The listing builds one solid part. Answer for the finished solid, in the listing's coordinates (mm). Face numbers are marked on the shaded views. A direction names the side the tool comes from. Give positions to 0.01 mm unless a question says otherwise; leave off trailing zeros. Order: outer loops, then holes, each group sorted by start corner. A loop starts at its lowest first (then second) coordinate and runs counter-clockwise, first axis right, second up.
```python
from build123d import *

# Parameters (mm, degrees)
EXTRUDE_1_DEPTH      = 25
CUT_EXTRUDE_1_REACH  = 113.383
SKETCH_2_R           = 3.2
CUT_EXTRUDE_2_REACH  = 113.383
SKETCH_3_R           = 3.2
SKETCH_14_W          = 22.5
SKETCH_14_H          = 2.5
SKETCH_14_W_2        = 2.5
SKETCH_14_H_2        = 22.5
CUT_EXTRUDE_12_DEPTH = 25
SKETCH_5_W           = 20.4
SKETCH_5_H           = 20.4
CUT_EXTRUDE_7_DEPTH  = 25
EXTRUDE_2_DEPTH      = 10
SKETCH_10_R          = 3.2
CUT_EXTRUDE_8_DEPTH  = 17.1
SKETCH_11_R          = 5.25
CUT_EXTRUDE_9_DEPTH  = 12.1
SKETCH_12_R          = 3.2
CUT_EXTRUDE_10_DEPTH = 17.1
SKETCH_13_R          = 5.25
CUT_EXTRUDE_11_DEPTH = 12.1
FILLET_2_R           = 2.5
FILLET_3_R           = 15
FILLET_5_R           = 2.5


with BuildPart() as part:
    # 스케치1 → 보스-돌출1 (new body)
    with BuildSketch(Plane(origin=(0, 0, 0), x_dir=(1, 0, 0), z_dir=(0, 1, 0))):
        Polygon((-17.5, 67.5), (-11.25, 67.5), (-11.25, 37.5), (11.25, 37.5), (11.25, 67.5), (17.5, 67.5), (17.5, -17.5), (-67.5, -17.5), (-67.5, -11.25), (-37.5, -11.25), (-37.5, 11.25), (-67.5, 11.25), (-67.5, 17.5), (-17.5, 17.5), align=None)
    extrude(amount=EXTRUDE_1_DEPTH)

    # 컷-돌출1: up to this face of the body (flat: up to its plane)
    cut_extrude_1_end = Plane(part.part.faces().sort_by_distance((-17.5, 12.5, -42.5))[0])
    # 스케치2 → 컷-돌출1 (cut, up to the picked face)
    with BuildSketch(Plane(origin=(17.5, 0, 0), x_dir=(0, 0, -1), z_dir=(1, 0, 0)), mode=Mode.PRIVATE) as cut_extrude_1_sk1:
        with Locations((60, 12.5)):
            Circle(SKETCH_2_R)
    cut_extrude_1_tool1 = split(extrude(cut_extrude_1_sk1.sketch, amount=-CUT_EXTRUDE_1_REACH, mode=Mode.PRIVATE), bisect_by=cut_extrude_1_end, keep=Keep.BOTH, mode=Mode.PRIVATE)
    # 스케치2 → 컷-돌출1 (cut, up to the picked face)
    with BuildSketch(Plane(origin=(17.5, 0, 0), x_dir=(0, 0, -1), z_dir=(1, 0, 0)), mode=Mode.PRIVATE) as cut_extrude_1_sk2:
        with Locations((45, 12.5)):
            Circle(SKETCH_2_R)
    cut_extrude_1_tool2 = split(extrude(cut_extrude_1_sk2.sketch, amount=-CUT_EXTRUDE_1_REACH, mode=Mode.PRIVATE), bisect_by=cut_extrude_1_end, keep=Keep.BOTH, mode=Mode.PRIVATE)
    add(cut_extrude_1_tool1.solids().sort_by(Axis((17.5, 12.5, -60), (-1, 0, 0)))[0], mode=Mode.SUBTRACT)
    add(cut_extrude_1_tool2.solids().sort_by(Axis((17.5, 12.5, -45), (-1, 0, 0)))[0], mode=Mode.SUBTRACT)

    # 컷-돌출2: up to this face of the body (flat: up to its plane)
    cut_extrude_2_end = Plane(part.part.faces().sort_by_distance((-42.5, 12.5, -17.5))[0])
    # 스케치3 → 컷-돌출2 (cut, up to the picked face)
    with BuildSketch(Plane.XY.offset(17.5), mode=Mode.PRIVATE) as cut_extrude_2_sk1:
        with Locations((-60, 12.5)):
            Circle(SKETCH_3_R)
    cut_extrude_2_tool1 = split(extrude(cut_extrude_2_sk1.sketch, amount=-CUT_EXTRUDE_2_REACH, mode=Mode.PRIVATE), bisect_by=cut_extrude_2_end, keep=Keep.BOTH, mode=Mode.PRIVATE)
    # 스케치3 → 컷-돌출2 (cut, up to the picked face)
    with BuildSketch(Plane.XY.offset(17.5), mode=Mode.PRIVATE) as cut_extrude_2_sk2:
        with Locations((-45, 12.5)):
            Circle(SKETCH_3_R)
    cut_extrude_2_tool2 = split(extrude(cut_extrude_2_sk2.sketch, amount=-CUT_EXTRUDE_2_REACH, mode=Mode.PRIVATE), bisect_by=cut_extrude_2_end, keep=Keep.BOTH, mode=Mode.PRIVATE)
    add(cut_extrude_2_tool1.solids().sort_by(Axis((-60, 12.5, 17.5), (0, 0, -1)))[0], mode=Mode.SUBTRACT)
    add(cut_extrude_2_tool2.solids().sort_by(Axis((-45, 12.5, 17.5), (0, 0, -1)))[0], mode=Mode.SUBTRACT)

    # 스케치14 → 컷-돌출12 (cut)
    with BuildSketch(Plane(origin=(0, 25, 0), x_dir=(1, 0, 0), z_dir=(0, 1, 0))):
        with Locations((0, 36.25)):
            Rectangle(SKETCH_14_W, SKETCH_14_H)
        with Locations((-36.25, 0)):
            Rectangle(SKETCH_14_W_2, SKETCH_14_H_2)
    extrude(amount=-CUT_EXTRUDE_12_DEPTH, mode=Mode.SUBTRACT)

    # 스케치5 → 컷-돌출7 (cut)
    with BuildSketch(Plane(origin=(0, 25, 0), x_dir=(1, 0, 0), z_dir=(0, 1, 0))):
        with Locations((-18.75, 18.75)):
            Rectangle(SKETCH_5_W, SKETCH_5_H)
        Polygon((-28.95, -8.55), (-28.95, -17.5), (17.5, -17.5), (17.5, 28.95), (8.55, 28.95), (8.55, -8.55), align=None)
    extrude(amount=-CUT_EXTRUDE_7_DEPTH, mode=Mode.SUBTRACT)

    # 스케치15 → 보스-돌출2 (add)
    with BuildSketch(Plane.XZ):
        Polygon((8.55, 8.55), (8.55, -28.95), (-8.55, -28.95), (-8.55, -8.55), (-28.95, -8.55), (-28.95, 8.55), align=None)
    extrude(amount=EXTRUDE_2_DEPTH)

    # 스케치10 → 컷-돌출8 (cut)
    with BuildSketch(Plane.XY.offset(8.55)):
        with Locations((-18.95, 15)):
            Circle(SKETCH_10_R)
        with Locations((-18.95, 0)):
            Circle(SKETCH_10_R)
    extrude(amount=-CUT_EXTRUDE_8_DEPTH, mode=Mode.SUBTRACT)

    # 스케치11 → 컷-돌출9 (cut)
    with BuildSketch(Plane.XY.offset(8.55)):
        with Locations((-18.95, 15)):
            Circle(SKETCH_11_R)
        with Locations((-18.95, 0)):
            Circle(SKETCH_11_R)
    extrude(amount=-CUT_EXTRUDE_9_DEPTH, mode=Mode.SUBTRACT)

    # 스케치12 → 컷-돌출10 (cut)
    with BuildSketch(Plane(origin=(8.55, 0, 0), x_dir=(0, 0, -1), z_dir=(1, 0, 0))):
        with Locations((18.95, 15)):
            Circle(SKETCH_12_R)
        with Locations((18.95, 0)):
            Circle(SKETCH_12_R)
    extrude(amount=-CUT_EXTRUDE_10_DEPTH, mode=Mode.SUBTRACT)

    # 스케치13 → 컷-돌출11 (cut)
    with BuildSketch(Plane(origin=(8.55, 0, 0), x_dir=(0, 0, -1), z_dir=(1, 0, 0))):
        with Locations((18.95, 15)):
            Circle(SKETCH_13_R)
        with Locations((18.95, 0)):
            Circle(SKETCH_13_R)
    extrude(amount=-CUT_EXTRUDE_11_DEPTH, mode=Mode.SUBTRACT)

    # 필렛2
    fillet_2_edges = [part.edges().sort_by_distance(p)[0] for p in [
        (-17.5, 12.5, -28.95),
        (-28.95, 12.5, -17.5),
        (-28.95, 12.5, 17.5),
        (17.5, 12.5, -28.95),
        (-10.2, -10, 8.55),
        (-28.95, -10, 0),
        (0, -10, -28.95),
        (8.55, -10, -10.2),
        (-17.5, 12.5, -67.5),
        (17.5, 12.5, -67.5),
        (-67.5, 12.5, 17.5),
        (-67.5, 12.5, -17.5),
    ]]
    fillet(fillet_2_edges, radius=FILLET_2_R)

    # 필렛3
    # the kernel refuses this fillet: 15 mm, written as the material it takes off along each edge
    with BuildSketch(Plane(origin=(-6.45, -10, -6.45), x_dir=(1, 0, 0), z_dir=(0, 0, -1))) as fillet_3_piece_1:
        with BuildLine():
            CenterArc((12.5, -2.5), 2.5, 0, 90)
            Line((15, -2.5), (15, 0))
            Line((15, 0), (12.5, 0))
        make_face()
    revolve(axis=Axis((-6.45, -10, -6.45), (0, -1, 0)), revolution_arc=90, mode=Mode.SUBTRACT)
    with BuildSketch(Plane(origin=(8.55, -10, 8.55), x_dir=(0, 0, -1), z_dir=(0, 1, 0))) as fillet_3_piece_2:
        with BuildLine():
            CenterArc((FILLET_3_R, FILLET_3_R), FILLET_3_R, 180, 90)
            Line((0, FILLET_3_R), (0, 0))
            Line((0, 0), (FILLET_3_R, 0))
        make_face()
    extrude(amount=72.5, mode=Mode.SUBTRACT)

    # 필렛5
    fillet_5_edges = [part.edges().sort_by_distance(p)[0] for p in [
        (-28.95, 0, 0),
        (0, 0, -28.95),
    ]]
    fillet(fillet_5_edges, radius=FILLET_5_R)


solid = part.part
```
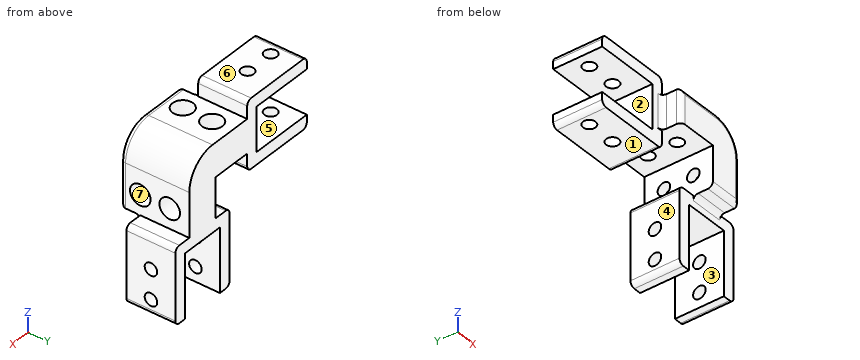
1) Find section D-D (y = 17). Count the separate pieces of the cut face and the enclosed holes in it, then the cut area to 3 significant figures.
Geometry says:
separate pieces: 3
enclosed holes: 0
area: 1,880 mm2
2) Straight lines are drawn through the part: probe 1 along Y at (x, z) = (-60, -12); probe 2 along Y at (x, z) = (6, -18.95); probe 3 along X at (y, z) = (21.5, -43). For each, find the intervals that lie inside material, in ascending order.
Geometry says:
probe 1: y = 0 to 9.3, 15.7 to 25
probe 2: y = -10 to -5.25, 5.25 to 9.75, 20.25 to 25
probe 3: x = -17.5 to -11.25, 11.25 to 17.5
3) Find section A-A (x = -60). Write down the section's boundary in (y, z), then the cut area to 4 significant figures.
Geometry says:
outline: (0, -17.5) - (9.3, -17.5) - (9.3, -11.25) - (0, -11.25) - close; (0, 11.25) - (9.3, 11.25) - (9.3, 17.5) - (0, 17.5) - close; (15.7, -17.5) - (25, -17.5) - (25, -11.25) - (15.7, -11.25) - close; (15.7, 11.25) - (25, 11.25) - (25, 17.5) - (15.7, 17.5) - close
area: 232.5 mm2
4) Find section C-C (x = -18.95). Write down the section's boundary in (y, z).
Geometry says:
outline: (-10, -8.55) - (-3.2, -8.55) - (-3.2, -3.55) - (-5.25, -3.55) - (-5.25, 8.55) - (-7.5, 8.55) arc R2.5 ccw to (-10, 6.05) - close; (3.2, -8.55) - (11.8, -8.55) - (11.8, -3.55) - (9.75, -3.55) - (9.75, 8.55) - (5.25, 8.55) - (5.25, -3.55) - (3.2, -3.55) - close; (18.2, -8.55) - (25, -8.55) - (25, 8.55) - (20.25, 8.55) - (20.25, -3.55) - (18.2, -3.55) - close
5) For a pull along Z with two mould halves and no side action, classify the marked faces 4, 5, 6 and 7 as +Z half, -Z half, draft (parallel to the pull), parting line (faces both ways), or undercut.
Geometry says:
face 4: draft
face 5: undercut
face 6: +Z half
face 7: undercut
6) Given P1, Ø17, axis at x = -18.95, y = 15, coming from the +Z side; P2, Ø4, axis at y = 12.5, z = -60, coming from the +X side; P3, Ø7, axis at y = 14, z = -12, coming from the +X side; P4, Ø6, axis at y = 9, z = 0.5, coming from the -X side, each flat-ended and moving along its own axis, determine where each tip first touches the part or whether it passes through.
Geometry says:
P1: stops at z = 8.55
P2: passes through
P3: stops at x = 8.55
P4: stops at x = -35
7) Find section B-B (z = -45). Write down the section's boundary in (x, y).
Geometry says:
outline: (-17.5, 0) - (-11.25, 0) - (-11.25, 9.3) - (-17.5, 9.3) - close; (-17.5, 15.7) - (-11.25, 15.7) - (-11.25, 25) - (-17.5, 25) - close; (11.25, 0) - (17.5, 0) - (17.5, 9.3) - (11.25, 9.3) - close; (11.25, 15.7) - (17.5, 15.7) - (17.5, 25) - (11.25, 25) - close
8) A tool of negligible diameter and unlimited length cuts with its end or side. For the marked faces 1, 2 and 3, from which of +Z, -Z, +X, -X, +Y, -Y can it reach the whole face along a straight path? Write none if from no direction.
Geometry says:
face 1: -Z, -X, +Y, -Y
face 2: -X, +Y, -Y
face 3: -Z, +Y, -Y
